Could you check a few things on this model? Use its own coordinates, in mm. A direction names the side the tool comes from. Give positions to 0.01 mm unless a question says otherwise; leave off trailing zeros. Write each loop counter-clockwise with the first axis right and the second up, starting at its lowest first coordinate (ties: lowest second). Pieces come first, ordered by that corner, then holes. Notation, with made-up numbers: (21, 0.5) -> (43, 0.5) arc R35 cw to (43, 37.5) -> close; hole circle Ø4 at (11.5, 17.25). An arc over 180 degrees is marked (long way). Write item = value, one per line. Start each with the question number.
```python
from build123d import *

# Parameters (mm, degrees)
F1_DEPTH = 101.6
F3_DEPTH = 152.4


with BuildPart() as f1:
    # F0 (on Top) → F1 (new body)
    with BuildSketch(Plane.XY):
        with BuildLine():
            ThreePointArc((471.423321, -25.710636), (139.580084, 2.415757), (0.027949, 304.8))
            Line((0.027949, 304.8), (-15.201777, 305.623494))
            ThreePointArc((-15.201777, 305.623494), (130.974786, -10.163429), (477.706076, -39.597778))
            Line((477.706076, -39.597778), (471.423321, -25.710636))
        make_face()
    extrude(amount=F1_DEPTH)

    # F2 (on face) → F3 (cut)
    with BuildSketch(Plane(origin=(381.67117, 172.673839, 0), x_dir=(-0.412194, 0.911096, 0), z_dir=(0.911096, 0.412194, 0))):
        Polygon((-139.049853, 76.2), (-316.849853, 76.2), (-316.849853, 25.4), (-232.984855, 25.4), (-139.049853, 25.4), align=None)
    extrude(amount=-F3_DEPTH, mode=Mode.SUBTRACT)


solid = f1.part
```
(1) Imagine slicing it at A-A (x = 361). Please give me the cut outline in (y, z), then the cut area to 3 significant figures.
(2) Imagine slicing it at C-C (z = 13.5). Please give me the cut outline in (x, y), then the cut area to 3 significant figures.
(3) I'm going to push flat-ended pins straight in: pin 1 (4 mm diameter, centred on y = 48.5, z = 13, fed in from +X); pin 2 (12 mm diameter, centred on y = 208, z = 88, fed in from -X); pin 3 (5 mm diameter, centred on x = 375.5, z = 84.5, fed in from +Y). Where does each tip first touch, or does it pass through?
(4) Imagine slicing it at B-B (y = 273.5). Please give me the cut outline in (x, z), then the cut area to 3 significant figures.
(5) If I drill on line 1 along Z through (x, y) = (384, -57); line 2 along Y through (x, z) = (332, 24); line 3 along X through (y, z) = (266, 68), over which ranges is the centre line in solid material (lowest first)? Write a range as from..to.
(6) On a 3-axis mill with a long thin cutter (end or side, diameter ignored), from which of +Z, -Z, +X, -X, +Y, -Y can I reach the whole of each face in a straight line? I mean faces 1 (the flat face through (156, -9, 0)), 2 (the flat face through (322.021, -65.206, 51.156)). Say none if no direction works.
(7) We'd pull the mould along Y, two halves only. Please class faces 3 (the flat face through (401, -53, 76.2)), 4 (the flat face through (474.61, -32.75, 88.72)): released by +Y, released by -Y, zero draft, split by the parting line, or undercut.
Answers below:
q1.outline = (-71.41, 0) -> (-56.1, 0) -> (-56.1, 25.4) -> (-71.41, 25.4) -> close; (-71.41, 76.2) -> (-56.1, 76.2) -> (-56.1, 101.6) -> (-71.41, 101.6) -> close
q1.area = 778 mm^2
q2.outline = (-15.2, 305.62) arc R346.36 ccw to (477.71, -39.6) -> (471.42, -25.71) arc R331.12 cw to (0.03, 304.8) -> close
q2.area = 10,900 mm^2
q3.pin_1 = 88.64
q3.pin_2 = -11.54
q3.pin_3 = -54.04
q4.outline = (-16.69, 0) -> (-1.45, 0) -> (-1.45, 101.6) -> (-16.69, 101.6) -> close
q4.area = 1,550 mm^2
q5.line_1 = 0..25.4, 76.2..101.6
q5.line_2 = -72.82..-57.58
q5.line_3 = -16.61..-1.37
q6.face_1 = -Z, +X, -X, +Y, -Y
q6.face_2 = +X, +Y
q7.face_3 = zero draft
q7.face_4 = released by +Y
